The listing builds one solid part. Answer for the finished solid, in the listing's coordinates (mm). A direction names the side the tool comes from. Give positions to 0.01 mm unless a question says otherwise; leave off trailing zeros. Order: outer loops, then holes, each group sorted by start corner. A loop starts at its lowest first (then second) coordinate and runs counter-clockwise, first axis right, second up.
```python
from build123d import *

# Parameters (mm, degrees)
SKETCH1_W           = 63.5
SKETCH1_H           = 50.8
BOSS_EXTRUDE1_DEPTH = 50.8
BOSS_EXTRUDE2_DEPTH = 50.8
SKETCH3_R           = 9.652
CUT_EXTRUDE2_DEPTH  = 6.35
BOSS_EXTRUDE3_DEPTH = 63.5
SKETCH6_R           = 9.652
CUT_EXTRUDE4_DEPTH  = 6.35
SKETCH7_R           = 5.715
CUT_EXTRUDE6_DEPTH  = 12.7


with BuildPart() as part:
    # Sketch1 → Boss-Extrude1 (new body)
    with BuildSketch(Plane(origin=(0, 0, 0), x_dir=(1, 0, 0), z_dir=(0, 1, 0))):
        Rectangle(SKETCH1_W, SKETCH1_H)
    extrude(amount=BOSS_EXTRUDE1_DEPTH)

    # Sketch2 → Boss-Extrude2 (add)
    with BuildSketch(Plane.XY.offset(25.4)):
        Polygon((63.5, 6.35), (31.75, 24.680871047), (31.75, 0), (63.5, 0), align=None)
    extrude(amount=-BOSS_EXTRUDE2_DEPTH)

    # Sketch3 → Cut-Extrude2 (cut)
    with BuildSketch(Plane(origin=(18.624630657, 32.25880657, 0), x_dir=(0.866025404, -0.5, 0), z_dir=(0.5, 0.866025404, 0))):
        with Locations((34.289443039, 0)):
            Circle(SKETCH3_R)
    extrude(amount=-CUT_EXTRUDE2_DEPTH, mode=Mode.SUBTRACT)

    # Sketch5 → Boss-Extrude3 (add, through all)
    with BuildSketch(Plane(origin=(31.75, 0, 0), x_dir=(0, 0, -1), z_dir=(1, 0, 0))):
        Polygon((-25.4, 50.8), (-66.802, 26.896544155), (-60.452, 15.898021527), (-25.4, 36.135303163), align=None)
    extrude(amount=-BOSS_EXTRUDE3_DEPTH)

    # Sketch6 → Cut-Extrude4 (cut)
    with BuildSketch(Plane(origin=(0, 49.098522628, 28.347045256), x_dir=(1, 0, 0), z_dir=(0, 0.866025404, 0.5))):
        with Locations((0, -20.500501101)):
            Circle(SKETCH6_R)
    extrude(amount=-CUT_EXTRUDE4_DEPTH, mode=Mode.SUBTRACT)

    # Sketch7 → Cut-Extrude6 (cut)
    with BuildSketch(Plane(origin=(0, 50.8, 0), x_dir=(1, 0, 0), z_dir=(0, 1, 0))):
        with Locations((-15.24, -10.16)):
            Circle(SKETCH7_R)
        with Locations((-15.24, 8.89)):
            Circle(SKETCH7_R)
        with Locations((16.51, -10.16)):
            Circle(SKETCH7_R)
        with Locations((16.51, 8.89)):
            Circle(SKETCH7_R)
    extrude(amount=-CUT_EXTRUDE6_DEPTH, mode=Mode.SUBTRACT)


solid = part.part
```
1) Find section B-B (x = -15.24). Write down the section's boundary in (y, z) (3 decimals), then the cut area to 3 significant figures.
Geometry says:
outline: (0, -25.4) - (50.8, -25.4) - (50.8, -14.605) - (38.1, -14.605) - (38.1, -3.175) - (50.8, -3.175) - (50.8, 4.445) - (38.1, 4.445) - (38.1, 15.875) - (50.8, 15.875) - (50.8, 25.4) - (26.897, 66.802) - (15.898, 60.452) - (36.135, 25.4) - (0, 25.4) - close
area: 2,850 mm2
2) A tool of negligible diameter and unlimited length cuts with its end or side. For faces 1 (the flat face through (45, 9.7, -0.1)), 2 (the flat face through (-15, 38.1, 10)), 3 (the flat face through (0, 50.8, 0)), from which of +Z, -Z, +X, -X, +Y, -Y can it reach the whole face along a straight path? Write none if from no direction.
Geometry says:
face 1: none
face 2: +Y
face 3: +Z, -Z, +X, -X, +Y
3) For a pull along Z with two mould halves and no side action, classify faces 4 (the flat face through (63.5, 3, 0)), 5 (the flat face through (0.444, 25.875, 43.171)), 6 (the flat face through (0.444, 33.704, 55.012)) as +Z half, -Z half, draft (parallel to the pull), parting line (faces both ways), or undercut.
Geometry says:
face 4: draft
face 5: undercut
face 6: +Z half
4) Find section C-C (x = 26). Write down the section's boundary in (y, z), then the cut area to 3 significant figures.
Geometry says:
outline: (0, -25.4) - (50.8, -25.4) - (50.8, 25.4) - (26.9, 66.8) - (15.9, 60.45) - (36.14, 25.4) - (0, 25.4) - close
area: 3,140 mm2
5) Straight lines are drawn through the part: probe 1 along X at (y, z) = (41, 10.16) (3 decimals); probe 2 along Z at (x, y) = (-15, 45); probe 3 along Z at (x, y) = (16, 42). For each, find the intervals that lie inside material, in ascending order.
Geometry says:
probe 1: x = -31.75 to -20.955, -9.525 to 10.795, 22.225 to 31.75
probe 2: z = -25.4 to -14.6, -3.18 to 4.45, 15.87 to 35.45
probe 3: z = -25.4 to -14.58, -3.2 to 4.47, 15.85 to 40.64
6) Given P1, Ø3.5, axis at x = -17.5, z = -10, coming from the +Y side; P2, Ø1, axis at y = 7.5, z = 26.5, coming from the -X side; P3, Ø3, axis at y = 12.5, z = 6, coming from the +X side, each flat-ended and moving along its own axis, determine where each tip first touches the part or whether it passes through.
Geometry says:
P1: stops at y = 38.1
P2: passes through
P3: stops at x = 55.45
7) Find section D-D (z = 59). Write down the section's boundary in (x, y), then the cut area to 3 significant figures.
Geometry says:
outline: (-31.75, 16.74) - (31.75, 16.74) - (31.75, 31.4) - (-31.75, 31.4) - close
area: 931 mm2
8) Find section A-A (y = 22). Write down the section's boundary in (x, z).
Geometry says:
outline: (-31.75, -25.4) - (36.39, -25.4) - (36.39, 25.4) - (-31.75, 25.4) - close; (-31.75, 49.88) - (31.75, 49.88) - (31.75, 63.97) - (-31.75, 63.97) - close
